Input: part model. Units: mm. Frame: model coordinates. A direction names the side the tool comes from. Give positions to 0.01 mm unless a question says otherwise; leave off trailing zeros. Loops run counter-clockwise (first coordinate to the right, second up) from the corner with the lowest first, then second, coordinate; pieces in that order, holes last. Notation, with made-up numbers: (-15, 35.25) -> (-9, 35.25) arc R20 cw to (-9, 57.25) -> close; hole circle Ø4 at (-23, 84.25). An arc over 180 degrees is marked (long way). Answer as a JSON object with one key per item and string values.
```python
from build123d import *

# Parameters (mm, degrees)
SKETCH1_R           = 7
BOSS_EXTRUDE1_DEPTH = 2.5
SKETCH2_R           = 4.5
BOSS_EXTRUDE2_DEPTH = 16
SKETCH3_R           = 1
CUT_EXTRUDE1_DEPTH  = 5


with BuildPart() as part:
    # Sketch1 → Boss-Extrude1 (new body)
    with BuildSketch(Plane.XY):
        Circle(SKETCH1_R)
    extrude(amount=BOSS_EXTRUDE1_DEPTH)

    # Sketch2 → Boss-Extrude2 (add)
    with BuildSketch(Plane.XY.offset(2.5)):
        Circle(SKETCH2_R)
    extrude(amount=BOSS_EXTRUDE2_DEPTH)

    # Sketch3 → Cut-Extrude1 (cut)
    with BuildSketch(Plane.XY.offset(18.5)):
        with Locations((0, 2.5)):
            Circle(SKETCH3_R)
        with Locations((2.5, 0)):
            Circle(SKETCH3_R)
        with Locations((0, -2.5)):
            Circle(SKETCH3_R)
        with Locations((-2.5, 0)):
            Circle(SKETCH3_R)
    extrude(amount=-CUT_EXTRUDE1_DEPTH, mode=Mode.SUBTRACT)


solid = part.part
```
Q1. Section D-D, the plane z = 4.75. Return the cut outline in (x, y).
Evaluation:
{"outline": "circle Ø9 at (0, 0)"}
Q2. Section C-C, the plane z = 14.5. Return the cut outline in (x, y), then the cut area to 3 significant figures.
Evaluation:
{"outline": "circle Ø9 at (0, 0); hole circle Ø2 at (-2.5, 0); hole circle Ø2 at (0, -2.5); hole circle Ø2 at (0, 2.5); hole circle Ø2 at (2.5, 0)", "area": "51.1 mm2"}
Q3. Draft query along Y for faces 3 (the cylindrical face through (-0.59, 4.46, 10.39)), 4 (the flat face through (0, -5, 2.5)), 5 (the cylindrical face through (-0.217, -3.476, 16.035)), 6 (the cylindrical face through (1.5, 0, 16)). Return one class per face: +Y half, -Y half, draft (parallel to the pull), parting line (faces both ways), or undercut.
Evaluation:
{"face 3": "parting line", "face 4": "draft", "face 5": "undercut", "face 6": "undercut"}
Q4. Access query for faces 1 (the flat face through (-3, 0, 13.5)), 2 (the flat face through (0, 0, 0)). Directions: +Z, -Z, +X, -X, +Y, -Y. A direction counts if a zero-diameter tool reaches every point of the face in a straight line with its end or side. Return the directions, or none.
Evaluation:
{"face 1": "+Z", "face 2": "-Z, +X, -X, +Y, -Y"}
Q5. Pin query (flat end, axial travel): pin 1 (1.8 mm diameter, centred on x = -2.5, y = 0, fed in from +Z); pin 2 (3 mm diameter, centred on y = -1, z = 4.5, fed in from +X); pin 3 (1.5 mm diameter, centred on x = -2, z = 13, fed in from -Y). Return the tip coordinate at first contact, or that it passes through.
Evaluation:
{"pin 1": "stops at z = 13.5", "pin 2": "stops at x = 4.5", "pin 3": "stops at y = -4.32"}
Q6. Ray query, line 1 along Y through (x, z) = (0, 16.25); line 2 along Z through (x, y) = (-4.5, 3.5); line 3 along Y through (x, z) = (-2.5, 16.25). Return the intervals inside material, ascending.
Evaluation:
{"line 1": "y = -4.5 to -3.5, -1.5 to 1.5, 3.5 to 4.5", "line 2": "z = 0 to 2.5", "line 3": "y = -3.74 to -1, 1 to 3.74"}
Q7. Section A-A, the plane y = 0. Return the cut outline in (x, z).
Evaluation:
{"outline": "(-7, 0) -> (7, 0) -> (7, 2.5) -> (4.5, 2.5) -> (4.5, 18.5) -> (3.5, 18.5) -> (3.5, 13.5) -> (1.5, 13.5) -> (1.5, 18.5) -> (-1.5, 18.5) -> (-1.5, 13.5) -> (-3.5, 13.5) -> (-3.5, 18.5) -> (-4.5, 18.5) -> (-4.5, 2.5) -> (-7, 2.5) -> close"}
